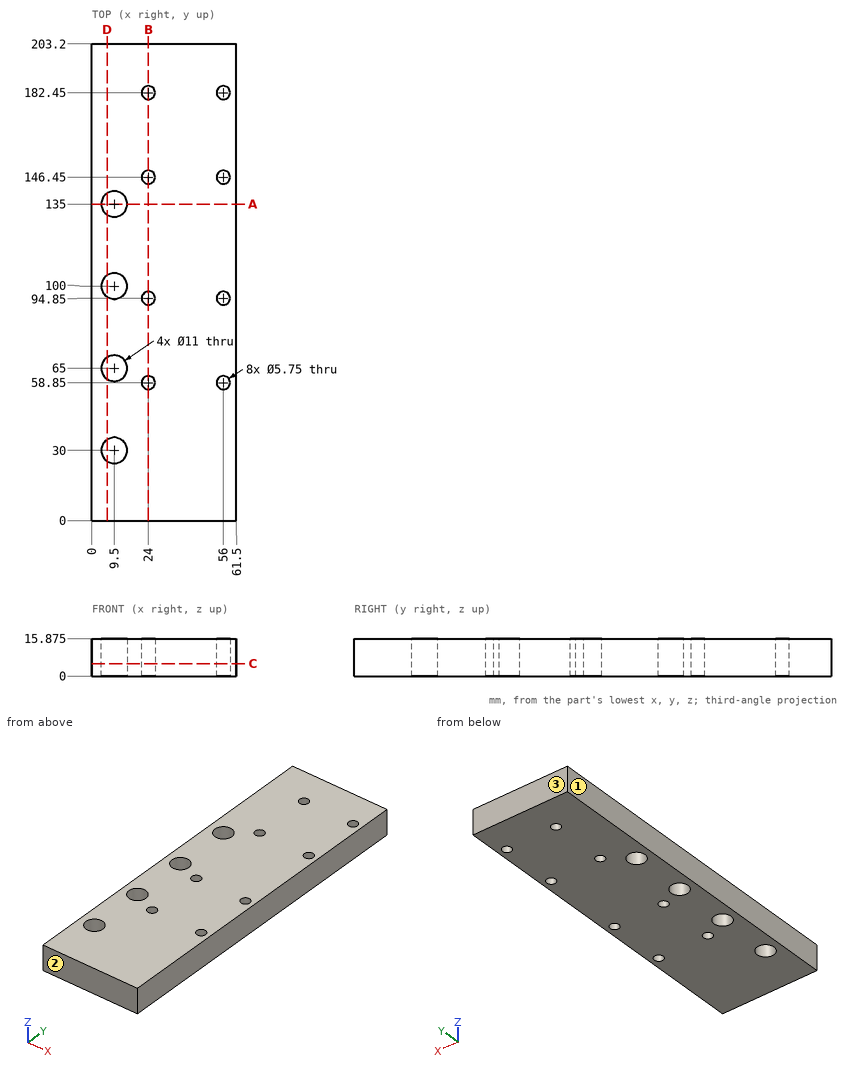
Study the drawing (mm; zero at the part's minimum x, y, z) and answer. Give positions to 0.01 mm unless a question says otherwise; leave off trailing zeros. Write each loop counter-clockwise with the first axis right and the second up, starting at its lowest first coordinate (ties: lowest second). Pieces come first, ordered by that corner, then holes. Notation, with made-up numbers: (-18.5, 10.5) -> (-5.5, 10.5) arc R20 cw to (-5.5, 28.5) -> close; hole circle Ø1 at (-33.5, -17). An arc over 180 degrees is marked (long way). Answer as a JSON object with one key per item and string values. Group by question number.
1) The mould has two halves that part along Y. Classify the marked faces 1, 2 and 3: +Y half, -Y half, draft (parallel to the pull), parting line (faces both ways), or undercut.
2) This flat-tipped pin is pushed along its axis until it touches: P1, Ø6.5, axis at x = 9.5, y = 30, coming from the -Z side (3 decimals). Where does it stop, or does it pass through?
3) Find section A-A (y = 135). Write down the section's boundary in (x, z) (3 decimals), and give its area (3 significant figures).
4) Find section B-B (x = 24). Write down the section's boundary in (y, z) (3 decimals), and give its area (3 significant figures).
5) Find section D-D (x = 6.5). Write down the section's boundary in (y, z) (3 decimals).
6) Consider L1, parallel to Y at x = 56, z = 6 (3 decimals); L2, parallel to X at y = 182.45, z = 12.25 (3 decimals); L3, parallel to Y at x = 25, z = 9.5. Determine where each line is inside the solid, lowest interval first. Write a range as from..to.
7) Find section C-C (z = 5.25). Count the separate pieces of the cut face and the enclosed holes in it, and give its area (3 significant figures).
Values follow:
{
 "1": {"face 1": "draft", "face 2": "-Y half", "face 3": "+Y half"},
 "2": {"P1": "passes through"},
 "3": {"outline": "(0, 0) -> (4, 0) -> (4, 15.875) -> (0, 15.875) -> close; (15, 0) -> (61.5, 0) -> (61.5, 15.875) -> (15, 15.875) -> close", "area": "802 mm2"},
 "4": {"outline": "(0, 0) -> (55.975, 0) -> (55.975, 15.875) -> (0, 15.875) -> close; (61.725, 0) -> (91.975, 0) -> (91.975, 15.875) -> (61.725, 15.875) -> close; (97.725, 0) -> (143.575, 0) -> (143.575, 15.875) -> (97.725, 15.875) -> close; (149.325, 0) -> (179.575, 0) -> (179.575, 15.875) -> (149.325, 15.875) -> close; (185.325, 0) -> (203.2, 0) -> (203.2, 15.875) -> (185.325, 15.875) -> close", "area": "2,860 mm2"},
 "5": {"outline": "(0, 0) -> (25.39, 0) -> (25.39, 15.875) -> (0, 15.875) -> close; (34.61, 0) -> (60.39, 0) -> (60.39, 15.875) -> (34.61, 15.875) -> close; (69.61, 0) -> (95.39, 0) -> (95.39, 15.875) -> (69.61, 15.875) -> close; (104.61, 0) -> (130.39, 0) -> (130.39, 15.875) -> (104.61, 15.875) -> close; (139.61, 0) -> (203.2, 0) -> (203.2, 15.875) -> (139.61, 15.875) -> close"},
 "6": {"L1": "y = 0..55.975, 61.725..91.975, 97.725..143.575, 149.325..179.575, 185.325..203.2", "L2": "x = 0..21.125, 26.875..53.125, 58.875..61.5", "L3": "y = 0..56.15, 61.55..92.15, 97.55..143.75, 149.15..179.75, 185.15..203.2"},
 "7": {"separate pieces": "1", "enclosed holes": "12", "area": "11,900 mm2"}
}
